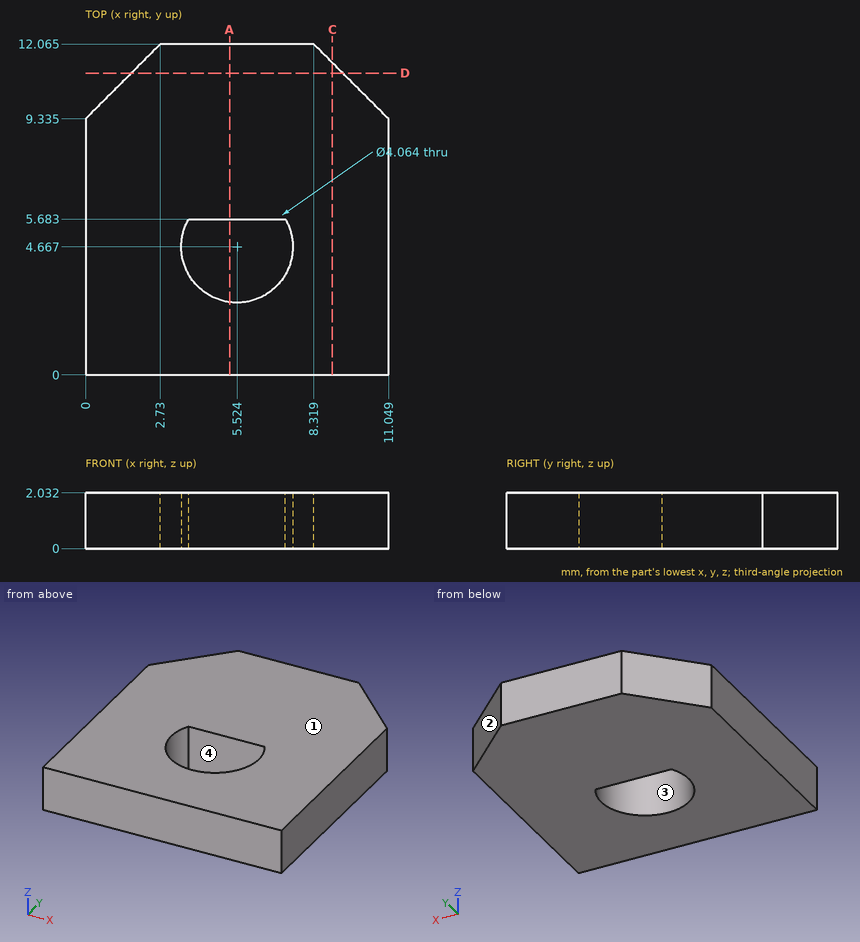
Check sheet for the drawn part. Datum: minimum x, y, z corner. Units: mm. Coordinates: 2 decimals unless noted, no trailing zeros. Loops run counter-clockwise (first coordinate to the right, second up) from the corner with the lowest first, then second, coordinate; pieces in that order, holes last. Notation, with made-up numbers: (-29.75, -7) -> (-25.75, -7) arc R31 cw to (-25.75, 20) -> close; hole circle Ø11 at (47.5, 62). An arc over 180 degrees is marked (long way). Answer in a Markdown table with one row per item.
1. Material ranges on line 1 along Y through (x, z) = (4, 0.75) (1 decimal); line 2 along X through (y, z) = (3.25, 0.3); line 3 along Y through (x, z) = (4.75, 1.95) (1 decimal), recorded low to high. Write a range as [from, to].
Check values:
| item | result |
|---|---|
| line 1 | y = [0, 3.3], [5.7, 12.1] |
| line 2 | x = [0, 4.07], [6.98, 11.05] |
| line 3 | y = [0, 2.8], [5.7, 12.1] |
2. Sectioned sample at D-D, the plane y = 11. Record the boundary of the cut face in (x, z) (1 decimal).
Check values:
| item | result |
|---|---|
| outline | (1.7, 0) -> (9.4, 0) -> (9.4, 2) -> (1.7, 2) -> close |
3. Sectioned sample at A-A, the plane x = 5.25. Record the boundary of the cut face in (y, z) (1 decimal).
Check values:
| item | result |
|---|---|
| outline | (0, 0) -> (2.7, 0) -> (2.7, 2) -> (0, 2) -> close; (5.7, 0) -> (12.1, 0) -> (12.1, 2) -> (5.7, 2) -> close |
4. Release check for a two-part mould opening along X. For the marked faces 1, 2, 3 and 4 record: released by +X, released by -X, zero draft, split by the parting line, or undercut.
Check values:
| item | result |
|---|---|
| face 1 | zero draft |
| face 2 | released by +X |
| face 3 | undercut |
| face 4 | undercut |
5. Sectioned sample at C-C, the plane x = 9. Record the boundary of the cut face in (y, z).
Check values:
| item | result |
|---|---|
| outline | (0, 0) -> (11.38, 0) -> (11.38, 2.03) -> (0, 2.03) -> close |
